from build123d import *

# Parameters (mm, degrees)
F0_R     = 6.25
F1_DEPTH = 38
F3_DEPTH = 15
F5_DEPTH = 23
F6_R     = 5.5
F7_DEPTH = 10
F7_TAPER = 23


with BuildPart() as f1:
    # F0 (on Front) → F1 (new body)
    with BuildSketch(Plane.XZ):
        Circle(F0_R)
    extrude(amount=F1_DEPTH)

    # F2 (on face) → F3 (cut)
    with BuildSketch(Plane.XZ.offset(38)):
        with BuildLine():
            Line((0, 1), (-2.2912878475, 1))
            ThreePointArc((-2.2912878475, 1), (0, -2.5), (2.2912878475, 1))
            Line((2.2912878475, 1), (0, 1))
        make_face()
    extrude(amount=-F3_DEPTH, mode=Mode.SUBTRACT)

    # F4 (on face) → F5 (cut)
    with BuildSketch(Plane(origin=(0, 0, 0), x_dir=(-1, 0, 0), z_dir=(0, 1, 0))):
        with BuildLine():
            Line((0, 1.5), (-2.3048861143, 1.5))
            ThreePointArc((-2.3048861143, 1.5), (0, -2.75), (2.3048861143, 1.5))
            Line((2.3048861143, 1.5), (0, 1.5))
        make_face()
    extrude(amount=-F5_DEPTH, mode=Mode.SUBTRACT)

    # F6 (on face) → F7 (cut)
    with BuildSketch(Plane(origin=(0, 0, 0), x_dir=(-1, 0, 0), z_dir=(0, 1, 0))):
        Circle(F6_R)
    extrude(amount=-F7_DEPTH, taper=F7_TAPER, mode=Mode.SUBTRACT)


solid = f1.part
For this review, take the finished solid that the model builds, in its own axes (mm). A direction names the side the tool comes from. Round coordinates to 2 decimals unless told otherwise and drop trailing zeros. Order: outer loops, then holes, each group sorted by start corner. A loop starts at its lowest first (then second) coordinate and runs counter-clockwise, first axis right, second up. Notation, with made-up numbers: (89.5, 37.25) -> (95.5, 37.25) arc R15 cw to (95.5, 41.25) -> close; hole circle Ø11 at (83, 63). An arc over 180 degrees is marked (long way). Write item = value, one per line. Start each with the question number.
1) Take a section at B-B on y = -11. State the section outline as (x, z) points.
2) Take a section at A-A on x = 0. State the section outline as (y, z) points, plus the area to 3 significant figures.
3) Tool access review of faces 1 (the face through (0.08, -14.62, -2.75)), 2 (the face through (-0.1, -30.6, -2.5)): name each direction out of +Z, -Z, +X, -X, +Y, -Y from which nothing blocks a thin tool from reaching the whole face with its end or side.
4) Insertion check: pin 1 (4 mm diameter, centred on y = -25.5, z = 3.5, fed in from +X); pin 2 (5 mm diameter, centred on x = 0, z = 0, fed in from +Y); pin 3 (6 mm diameter, centred on x = 5, y = -19, fed in from -Z). Each pin has a flat end and moves straight along its axis. Give the tip position at first contact, or say it passes through.
5) The part is to be moulded in two halves that separate along X. For faces 3 (the face through (0, -31, 1)), 4 (the face through (5.96, -18.73, 1.88)), 5 (the face through (0, 0, -6)), say which applies: +X half, -X half, draft (parallel to the pull), parting line (faces both ways), or undercut.
6) To check wall thickness, follow line 1 (Z direction, x = 0, y = -11.25); line 2 (Z direction, x = 0, y = -24); line 3 (X direction, y = -14, z = -1). State the ranges of each line that lie inside material, in increasing order. Write a range as from..to.
Verdict:
q1.outline = circle Ø12.5 at (0, 0); hole (-2.3, 1.5) arc R2.75 ccw (long way) to (2.3, 1.5) -> close
q2.outline = (-38, -6.25) -> (0, -6.25) -> (0, -5.5) -> (-6.48, -2.75) -> (-23, -2.75) -> (-23, -2.5) -> (-38, -2.5) -> close; (-38, 1) -> (-23, 1) -> (-23, 1.5) -> (-9.42, 1.5) -> (0, 5.5) -> (0, 6.25) -> (-38, 6.25) -> close
q2.area = 297 mm2
q3.face_1 = +Y
q3.face_2 = +Y, -Y
q4.pin_1 = 6.07
q4.pin_2 = -7.07
q4.pin_3 = -5.92
q5.face_3 = undercut
q5.face_4 = parting line
q5.face_5 = draft
q6.line_1 = -6.25..-2.75, 1.5..6.25
q6.line_2 = -6.25..-2.5, 1..6.25
q6.line_3 = -6.17..-2.56, 2.56..6.17
